Autodesk Inventor part; units mm, degrees
ref_plane "Work Plane3" through (10.8, 4.25, -2.5) normal (0, 0, -1) x (-1, 0, 0)
ref_plane "YZ Plane" through (0, 0, 0) normal (1, 0, 0) x (0, 1, 0)
ref_plane "XZ Plane" through (0, 0, 0) normal (0, 1, 0) x (-1, 0, 0)
sketch "Sketch1" plane through (0, 0, 0) normal (0, 0, 1) x (1, 0, 0)
  line L0 (-5, -2.5) -> (5, -2.5)
  line L1 (5, -2.5) -> (12.675, 0)
  line L2 (-5, -2.5) -> (-12.675, 0)
  line L3 (12.675, 0) -> (-12.675, 0) construction
  line L4 (12.675, 0) -> (12.675, 8.7)
  line L5 (-12.675, 0) -> (-12.675, 8.7)
  line L6 (-12.675, 8.7) -> (-4.75, 23.1)
  line L7 (-4.75, 23.1) -> (-4.75, 25.1)
  line L8 (-4.75, 25.1) -> (4.75, 25.1)
  line L9 (4.75, 25.1) -> (4.75, 23.1)
  line L10 (4.75, 23.1) -> (12.675, 8.7)
  line L11 (0, -8.02) -> (0, 30.62)
  line L12 (0, 25.1) -> (0, -2.5)
  point P0 (0, 0)
  point P1 (0, 0)
  dimension "d0" = 10
  dimension "d1" = 25.35
  dimension "d2" = 2.5
  dimension "d3" = 8.7
  dimension "d4" = 27.6
  dimension "d6" = 2
  dimension "d7" = 9.5
extrude "Body" add sketch "Sketch1" along normal blind 8.1 contours L11 L8 L9 L10 L4 L1 L0
sketch "Sketch5" plane through (0, 0, 0) normal (0, 0, -1) x (-1, 0, 0)
  circle A0 centre (-10.8, 4.25) radius 1.25
  line L0 (-10.8, 4.25) -> (0, 4.25) construction
  line L1 (0, 25.1) -> (0, -2.5)
  line L2 (0, -2.5) -> (-5, -2.5)
  point P0 (0, 0)
  dimension "d26" = 2.5
  dimension "d27" = 10.8
  dimension "d28" = 6.75
extrude "PinCylinder" add sketch "Sketch5" along normal blind 1
ref_plane "Work Plane3" through (10.8, 4.25, -2.5) normal (0, 0, -1) x (-1, 0, 0)
sketch "Sketch6" plane through (10.8, 4.25, -2.5) normal (0, 0, -1) x (-1, 0, 0)
  circle A0 centre (0, 0) radius 1.25
  circle A1 centre (0, 0) radius 0.75
  point P0 (10.8, -4.25)
  dimension "d32" = 1.5
loft "Loft2" add profiles "Sketch6" section 1 edges at (12.05, 4.25, -1) contours A1
sketch "Sketch7" plane through (0, 0, 0) normal (0, 0, -1) x (-1, 0, 0)
  line L0 (0, -0.7) -> (-4.15, -0.7)
  line L1 (-4.15, -0.7) -> (-4.15, 24.1)
  line L2 (0, -2.5) -> (-5, -2.5)
  line L3 (0, 25.1) -> (0, -2.5)
  line L4 (-4.15, 24.1) -> (0, 24.1)
  point P0 (0, 0)
  dimension "d37" = 4.15
  dimension "d38" = 24.8
  dimension "d39" = 1.8
extrude "MiddleCutout" cut sketch "Sketch7" against normal blind 1
mirror "Mirror1" about plane through (0, 25.1, 0) normal (-1, 0, 0)
properties part number "Inkjet"
Here's how the part is built. I have some questions about the finished solid (model axes, mm). A direction names the side the tool comes from. Give positions to 0.01 mm unless a question says otherwise; leave off trailing zeros. Order: outer loops, then holes, each group sorted by start corner. A loop starts at its lowest first (then second) coordinate and runs counter-clockwise, first axis right, second up. Notation, with made-up numbers: (9, -13) -> (30, -13) arc R19 ccw to (30, -9) -> close; hole circle Ø6 at (-14.5, -37.5). An arc over 180 degrees is marked (long way). Use a Markdown table: item, result. Add a question column.
Item 1: Imagine slicing it at D-D on x = 10.8. Please give me the cut outline in (y, z).
Item 2: For faces 4 (the face through (-10.223, 3.141, -0.493)), 5 (the face through (-4.75, 24, 4)), 6 (the face through (12.675, 4, 4)), 7 (the face through (4.75, 24, 4)), which set-ups out of +Z, -Z, +X, -X, +Y, -Y let a thin tool reach every point of the face, with its end or its side?
Item 3: Will these pins go through, and if not, where does the flat tip stop? pin 1 (1.5 mm diameter, centred on x = -7.5, z = 2, fed in from +Y); pin 2 (6 mm diameter, centred on x = -7, z = 0.5, fed in from +Y); pin 3 (1 mm diameter, centred on y = 11, z = 4.5, fed in from +X); pin 4 (4 mm diameter, centred on x = -2, y = 16.5, fed in from -Z).
Item 4: Imagine slicing it at A-A on z = 2.5. Please give me the cut outline in (x, y) (3 decimals).
Item 5: Imagine slicing it at C-C on z = -0.5. Please give me the cut outline in (x, y).
Item 6: I need wall thicknesses on line 1 (Z direction, x = 8.25, y = 12); line 2 (Z direction, x = 0, y = 20); line 3 (X direction, y = 8.75, z = 0.5). Which ranges of each line are inside material? Lowest first, please.
Item 7: Imagine slicing it at B-B on y = 1. Please give me the cut outline in (x, z) (3 decimals).
Item 8: If we mould it in two halves opening along X, with no side actions, what happens to faces 1 (the face through (0, 25.1, 4)), 2 (the face through (-9.976, 3.908, -2.073)), 3 (the face through (8.78, -1.27, 3.99))? For each: pulls with the +X half, pulls with the -X half, needs draft (parallel to the pull), parting line crosses it, or undercut.
Data:
| question | item | result |
|---|---|---|
| 1 | outline | (-0.61, 0) -> (3, 0) -> (3, -1) -> (3.5, -2.5) -> (5, -2.5) -> (5.5, -1) -> (5.5, 0) -> (12.11, 0) -> (12.11, 8.1) -> (-0.61, 8.1) -> close |
| 2 | face 4 | -Z |
| 2 | face 5 | +Z, -Z, -X, +Y |
| 2 | face 6 | +Z, -Z, +X, +Y, -Y |
| 2 | face 7 | +Z, -Z, +X, +Y |
| 3 | pin 1 | stops at y = 19.47 |
| 3 | pin 2 | stops at y = 25.1 |
| 3 | pin 3 | stops at x = 11.68 |
| 3 | pin 4 | stops at z = 1 |
| 4 | outline | (-12.675, 0) -> (-5, -2.5) -> (5, -2.5) -> (12.675, 0) -> (12.675, 8.7) -> (4.75, 23.1) -> (4.75, 25.1) -> (-4.75, 25.1) -> (-4.75, 23.1) -> (-12.675, 8.7) -> close |
| 5 | outline | circle Ø2.5 at (-10.8, 4.25); circle Ø2.5 at (10.8, 4.25) |
| 6 | line 1 | z = 0 to 8.1 |
| 6 | line 2 | z = 1 to 8.1 |
| 6 | line 3 | x = -12.65 to -4.15, 4.15 to 12.65 |
| 7 | outline | (-12.675, 0) -> (-4.15, 0) -> (-4.15, 1) -> (4.15, 1) -> (4.15, 0) -> (12.675, 0) -> (12.675, 8.1) -> (-12.675, 8.1) -> close |
| 8 | face 1 | needs draft |
| 8 | face 2 | undercut |
| 8 | face 3 | pulls with the +X half |
